Source: CAD feature listing. Evaluate the final solid. Frame: model axes, mm. A direction names the side the tool comes from. Coordinates: 2 decimals unless noted, no trailing zeros. Write each loop counter-clockwise with the first axis right and the second up, starting at its lowest first coordinate (ties: lowest second). Pieces come first, ordered by that corner, then holes. Notation, with made-up numbers: (62, 73.25) -> (74, 73.25) arc R16 ccw to (74, 102.25) -> close; hole circle Ø4 at (44.25, 2). An arc over 180 degrees is marked (long way). Write item = value, one per line.
from build123d import *

# Parameters (mm, degrees)
SKETCH1_W           = 25.4
SKETCH1_H           = 25.4
BOSS_EXTRUDE1_DEPTH = 50.8
SKETCH2_R           = 2.5527
CUT_EXTRUDE1_DEPTH  = 12.7
CUT_EXTRUDE2_START  = -12.7
SKETCH3_R           = 2.5527
CUT_EXTRUDE2_DEPTH  = 12.7
SKETCH4_R           = 3.175
CUT_EXTRUDE3_DEPTH  = 59.198711326


with BuildPart() as part:
    # Sketch1 → Boss-Extrude1 (new, symmetric)
    with BuildSketch(Plane.XY):
        Rectangle(SKETCH1_W, SKETCH1_H)
    extrude(amount=BOSS_EXTRUDE1_DEPTH, both=True)

    # Sketch2 → Cut-Extrude1 (cut)
    with BuildSketch(Plane.XY.offset(50.8)):
        Circle(SKETCH2_R)
    extrude(amount=-CUT_EXTRUDE1_DEPTH, mode=Mode.SUBTRACT)

    # Sketch3 → Cut-Extrude2 (cut)
    with BuildSketch(Plane(origin=(0, 0, -50.8), x_dir=(-1, 0, 0), z_dir=(0, 0, -1)).offset(CUT_EXTRUDE2_START)):
        with Locations(Location((0, 0, 0), (0, 0, 180))):
            Circle(SKETCH3_R)
    extrude(amount=CUT_EXTRUDE2_DEPTH, mode=Mode.SUBTRACT)

    # Sketch4 → Cut-Extrude3 (cut, through all)
    with BuildSketch(Plane(origin=(12.7, 0, 0), x_dir=(0, 0, -1), z_dir=(1, 0, 0))):
        with Locations((-31.75, 0)):
            Circle(SKETCH4_R)
        with Locations((31.75, 0)):
            Circle(SKETCH4_R)
    extrude(amount=-CUT_EXTRUDE3_DEPTH, mode=Mode.SUBTRACT)


solid = part.part
1) Cut plane D-D, the plane x = 8.75. Output: boundary loops of the cut face in (y, z) (3 decimals), and give its area (3 significant figures).
Answer block:
outline = (-12.7, -50.8) -> (12.7, -50.8) -> (12.7, 50.8) -> (-12.7, 50.8) -> close; hole circle Ø6.35 at (0, -31.75); hole circle Ø6.35 at (0, 31.75)
area = 2,520 mm2
2) Cut plane A-A, the plane z = 31.75. Output: boundary loops of the cut face in (x, y) (3 decimals).
Answer block:
outline = (-12.7, -12.7) -> (12.7, -12.7) -> (12.7, -3.175) -> (-12.7, -3.175) -> close; (-12.7, 3.175) -> (12.7, 3.175) -> (12.7, 12.7) -> (-12.7, 12.7) -> close
3) First-contact query: pin 1 Ø4 at (x, y) = (0, 0) entering from -Z; pin 2 Ø1.5 at (x, y) = (1, -1) entering from +Z. Flat tips, straight axial feed; report the tip coordinate or a pass-through.
Answer block:
pin_1 = -38.1
pin_2 = 38.1
4) Material intervals for probe 1 along Z at (x, y) = (0.75, -1.25); probe 2 along Z at (x, y) = (-3.5, -2.25); probe 3 along Y at (x, z) = (0, -43.75), sorted ascending. Write a range as [from, to].
Answer block:
probe_1 = [-38.1, -34.67], [-28.83, 28.83], [34.67, 38.1]
probe_2 = [-50.8, -33.99], [-29.51, 29.51], [33.99, 50.8]
probe_3 = [-12.7, -2.55], [2.55, 12.7]
5) Cut plane C-C, the plane x = 0. Output: boundary loops of the cut face in (y, z) (3 decimals), and give its area (3 significant figures).
Answer block:
outline = (-12.7, -50.8) -> (-2.553, -50.8) -> (-2.553, -38.1) -> (2.553, -38.1) -> (2.553, -50.8) -> (12.7, -50.8) -> (12.7, 50.8) -> (2.553, 50.8) -> (2.553, 38.1) -> (-2.553, 38.1) -> (-2.553, 50.8) -> (-12.7, 50.8) -> close; hole circle Ø6.35 at (0, -31.75); hole circle Ø6.35 at (0, 31.75)
area = 2,390 mm2
6) Cut plane B-B, the plane y = 0. Output: boundary loops of the cut face in (x, z) (3 decimals).
Answer block:
outline = (-12.7, -50.8) -> (-2.553, -50.8) -> (-2.553, -38.1) -> (2.553, -38.1) -> (2.553, -50.8) -> (12.7, -50.8) -> (12.7, -34.925) -> (-12.7, -34.925) -> close; (-12.7, -28.575) -> (12.7, -28.575) -> (12.7, 28.575) -> (-12.7, 28.575) -> close; (-12.7, 34.925) -> (12.7, 34.925) -> (12.7, 50.8) -> (2.553, 50.8) -> (2.553, 38.1) -> (-2.553, 38.1) -> (-2.553, 50.8) -> (-12.7, 50.8) -> close
7) Reachability of faces 4 (the cylindrical face through (2.435, -0.767, -44.361)), 5 (the flat face through (0, -12.7, 1)), 6 (the flat face through (0, 0, 38.1)) from +Z, -Z, +X, -X, +Y, -Y: full face, straight path, thin tool, end or side. Return the list, or none.
Answer block:
face_4 = -Z
face_5 = +Z, -Z, +X, -X, -Y
face_6 = +Z
8) Pull-direction query (Y, two-part tool) for faces 1 (the flat face through (0, 12.7, 1)), 2 (the flat face through (-12.7, 0, 1)), 3 (the cylindrical face through (0.18, 0.14, 34.92)); classes: +Y half, -Y half, draft (parallel to the pull), parting line (faces both ways), or undercut.
Answer block:
face_1 = +Y half
face_2 = draft
face_3 = undercut
